Check sheet for the modelled part. Datum: model origin and axes. Units: mm. Coordinates: 2 decimals unless noted, no trailing zeros. Loops run counter-clockwise (first coordinate to the right, second up) from the corner with the lowest first, then second, coordinate; pieces in that order, holes last.
```python
from build123d import *

# Parameters (mm, degrees)
SKETCH1_W           = 711.2
SKETCH1_H           = 127
BOSS_EXTRUDE1_DEPTH = 4.7625
SKETCH2_W           = 13.208
SKETCH2_H           = 51.308
CUT_EXTRUDE1_DEPTH  = 5.7625
SKETCH3_W           = 25.908
SKETCH3_H           = 5.2705
CUT_EXTRUDE2_DEPTH  = 5.7625


with BuildPart() as part:
    # Sketch1 → Boss-Extrude1 (new body)
    with BuildSketch(Plane(origin=(0, 0, 0), x_dir=(1, 0, 0), z_dir=(0, 1, 0))):
        with Locations((0, 63.5)):
            Rectangle(SKETCH1_W, SKETCH1_H)
    extrude(amount=BOSS_EXTRUDE1_DEPTH)

    # Sketch2 → Cut-Extrude1 (cut, through all)
    with BuildSketch(Plane(origin=(0, 0, 0), x_dir=(-1, 0, 0), z_dir=(0, -1, 0))):
        with Locations((-112.7125, 78.82990203)):
            Rectangle(SKETCH2_W, SKETCH2_H)
        with Locations((112.7125, 78.82990203)):
            Rectangle(SKETCH2_W, SKETCH2_H)
    extrude(amount=-CUT_EXTRUDE1_DEPTH, mode=Mode.SUBTRACT)

    # Sketch3 → Cut-Extrude2 (cut, through all)
    with BuildSketch(Plane.XZ):
        with Locations((-309.5625, -115.09375)):
            Rectangle(SKETCH3_W, SKETCH3_H)
        with Locations((-207.9625, -115.09375)):
            Rectangle(SKETCH3_W, SKETCH3_H)
        with Locations((207.9625, -115.09375)):
            Rectangle(SKETCH3_W, SKETCH3_H)
        with Locations((309.5625, -115.09375)):
            Rectangle(SKETCH3_W, SKETCH3_H)
    extrude(amount=-CUT_EXTRUDE2_DEPTH, mode=Mode.SUBTRACT)


solid = part.part
```
1) Section check B-B on y = 0.8. Enter the section's corners in (x, z), plus the area to 3 significant figures.
Answer sheet:
outline: (-355.6, -127) - (355.6, -127) - (355.6, 0) - (-355.6, 0) - close; hole (-322.52, -117.73) - (-296.61, -117.73) - (-296.61, -112.46) - (-322.52, -112.46) - close; hole (-220.92, -117.73) - (-195.01, -117.73) - (-195.01, -112.46) - (-220.92, -112.46) - close; hole (-119.32, -104.48) - (-106.11, -104.48) - (-106.11, -53.18) - (-119.32, -53.18) - close; hole (106.11, -104.48) - (119.32, -104.48) - (119.32, -53.18) - (106.11, -53.18) - close; hole (195.01, -117.73) - (220.92, -117.73) - (220.92, -112.46) - (195.01, -112.46) - close; hole (296.61, -117.73) - (322.52, -117.73) - (322.52, -112.46) - (296.61, -112.46) - close
area: 88,400 mm2
2) Scan lines: line 1 (X direction, y = 1.8, z = -80.5); line 2 (Z direction, x = -199, y = 3.7). Record each from-to range of solid material in increasing order.
Answer sheet:
line 1: x = -355.6 to -119.32, -106.11 to 106.11, 119.32 to 355.6
line 2: z = -127 to -117.73, -112.46 to 0
3) Section check A-A on x = -201. Enter the section's corners in (y, z), plus the area to 3 significant figures.
Answer sheet:
outline: (0, -127) - (4.76, -127) - (4.76, -117.73) - (0, -117.73) - close; (0, -112.46) - (4.76, -112.46) - (4.76, 0) - (0, 0) - close
area: 580 mm2
4) Section check C-C on z = -97.5. Enter the section's corners in (x, y), plus the area to 3 significant figures.
Answer sheet:
outline: (-355.6, 0) - (-119.32, 0) - (-119.32, 4.76) - (-355.6, 4.76) - close; (-106.11, 0) - (106.11, 0) - (106.11, 4.76) - (-106.11, 4.76) - close; (119.32, 0) - (355.6, 0) - (355.6, 4.76) - (119.32, 4.76) - close
area: 3,260 mm2
